```python
from build123d import *

# Parameters (mm, degrees)
SKETCH1_W           = 50.8
SKETCH1_H           = 25.4
BOSS_EXTRUDE1_DEPTH = 2.38125
SKETCH2_R           = 2.38125
CUT_EXTRUDE1_DEPTH  = 41.937805342
SKETCH3_R           = 2.38125
CUT_EXTRUDE2_DEPTH  = 41.937805342
CUT_EXTRUDE3_DEPTH  = 41.937805342
FILLET1_R           = 1.27


with BuildPart() as part:
    # Sketch1 → Boss-Extrude1 (new, symmetric)
    with BuildSketch(Plane.XY):
        with Locations((0, 19.05)):
            Rectangle(SKETCH1_W, SKETCH1_H)
        Polygon((25.4, 0), (0, 0), (0, -2.50825), (-25.4, -2.50825), (-25.4, -6.35), (25.4, -6.35), align=None)
        Polygon((-25.4, 6.35), (-25.4, 2.50825), (0, 2.50825), (0, 0), (25.4, 0), (25.4, 6.35), align=None)
    extrude(amount=BOSS_EXTRUDE1_DEPTH, both=True)

    # Sketch2 → Cut-Extrude1 (cut, through all)
    with BuildSketch(Plane.XY.offset(2.38125)):
        with Locations((20.47875, 0)):
            Circle(SKETCH2_R)
    extrude(amount=-CUT_EXTRUDE1_DEPTH, mode=Mode.SUBTRACT)

    # Sketch3 → Cut-Extrude2 (cut, through all)
    with BuildSketch(Plane.XY.offset(2.38125)):
        with Locations((-15.999222806, 25.4)):
            Circle(SKETCH3_R)
    extrude(amount=-CUT_EXTRUDE2_DEPTH, mode=Mode.SUBTRACT)

    # Sketch4 → Cut-Extrude3 (cut, through all)
    with BuildSketch(Plane.XY.offset(2.38125)):
        Polygon((-6.35, 31.75), (25.4, 6.35), (25.4, 31.75), align=None)
    extrude(amount=-CUT_EXTRUDE3_DEPTH, mode=Mode.SUBTRACT)

    # Fillet1
    fillet1_edges = [part.edges().sort_by_distance(p)[0] for p in [
        (-25.4, 31.75, 0),
        (25.4, -6.35, 0),
        (-25.4, -6.35, 0),
        (-25.4, 2.50825, 0),
        (-6.35, 31.75, 0),
        (25.4, 6.35, 0),
    ]]
    fillet(fillet1_edges, radius=FILLET1_R)


solid = part.part
```
Input: part model. Units: mm. Frame: model coordinates. A direction names the side the tool comes from. Round coordinates to 2 decimals unless told otherwise and drop trailing zeros. Order: outer loops, then holes, each group sorted by start corner. A loop starts at its lowest first (then second) coordinate and runs counter-clockwise, first axis right, second up. Notation, with made-up numbers: (-22.75, -1.75) - (8.25, -1.75) arc R27 ccw to (8.25, 29.25) - close; hole circle Ø1 at (88.5, -13.5). An arc over 180 degrees is marked (long way). One line per question, with ' | ' between items. Start each with the question number.
1) Set-up query: faces 1 (the cylindrical face through (22.75, 0.72, 0.03)), 2 (the flat face through (0, 0, 0)). Return all of +Z, -Z, +X, -X, +Y, -Y with unobstructed straight access to the full face (end or side cutting, diameter ignored); none if empty.
2) Contact query for flat-ended pins moving along their axis: P1, Ø4, axis at x = -16, y = 25.4, coming from the -Z side; P2, Ø2, axis at y = -1, z = -1, coming from the -X side. Output: stop coordinate, or through.
3) Cut plane A-A, the plane x = -20.5. Return the cut outline in (y, z), then the cut area to 3 significant figures.
4) Cut plane C-C, the plane y = 0. Return the cut outline in (x, z), then the cut area to 3 significant figures.
5) Cut plane B-B, the plane z = -1.45. Return the cut outline in (x, y), then the cut area to 3 significant figures.
6) Pull-direction query (Y, two-part tool) for faces 3 (the cylindrical face through (-25.018, -5.988, 0.033)), 4 (the flat face through (-13, -2.508, 0)), 5 (the cylindrical face through (25.27, 6.3, -0.03)); classes: +Y half, -Y half, draft (parallel to the pull), parting line (faces both ways), or undercut.
7) Ray query, probe 1 along Y at (x, z) = (-16.5, 1.65); probe 2 along Y at (x, z) = (-7, 0.2); probe 3 along Y at (x, z) = (19.5, 1.75). Return the intervals inside material, ascending.
8) Cut plane D-D, the plane x = 15. Return the cut outline in (y, z).
Worked out:
1) face 1: +Z, -Z | face 2: +Z, -Z, -X
2) P1: passes through | P2: stops at x = 0
3) outline: (-6.35, -2.38) - (-2.51, -2.38) - (-2.51, 2.38) - (-6.35, 2.38) - close; (2.51, -2.38) - (31.75, -2.38) - (31.75, 2.38) - (2.51, 2.38) - close | area: 158 mm^2
4) outline: (0, -2.38) - (18.1, -2.38) - (18.1, 2.38) - (0, 2.38) - close; (22.86, -2.38) - (25.4, -2.38) - (25.4, 2.38) - (22.86, 2.38) - close | area: 98.3 mm^2
5) outline: (-25.4, -5.08) arc R1.27 ccw to (-24.13, -6.35) - (24.13, -6.35) arc R1.27 ccw to (25.4, -5.08) - (25.4, 5.74) arc R1.27 ccw to (24.92, 6.73) - (-6, 31.47) arc R1.27 ccw to (-6.8, 31.75) - (-24.13, 31.75) arc R1.27 ccw to (-25.4, 30.48) - (-25.4, 3.78) arc R1.27 ccw to (-24.13, 2.51) - (0, 2.51) - (0, -2.51) - (-25.4, -2.51) - close; hole circle Ø4.76 at (-16, 25.4); hole circle Ø4.76 at (20.48, 0) | area: 1,370 mm^2
6) face 3: -Y half | face 4: undercut | face 5: +Y half
7) probe 1: y = -6.35 to -2.51, 2.51 to 23.07, 27.73 to 31.75 | probe 2: y = -6.35 to -2.51, 2.51 to 31.75 | probe 3: y = -6.35 to -2.17, 2.17 to 11.07
8) outline: (-6.35, -2.38) - (14.67, -2.38) - (14.67, 2.38) - (-6.35, 2.38) - close
